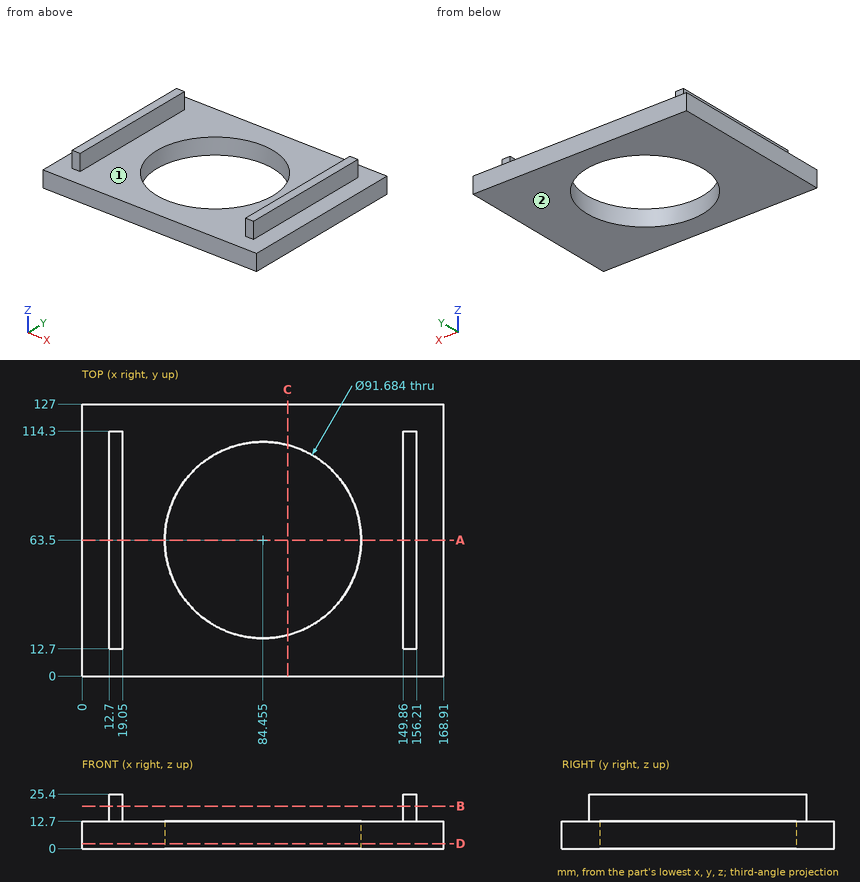
Can you work these out from the drawing? Everything is in mm from the part's minimum corner. Coordinates: 2 decimals unless noted, no trailing zeros. Write each loop counter-clockwise with the first axis right and the second up, starting at its lowest first coordinate (ties: lowest second). Pieces come first, ordered by that corner, then holes. Notation, with made-up numbers: (-13, 9.5) -> (38, 9.5) arc R27 cw to (38, 30.5) -> close; hole circle Ø4 at (21, 87.5). An arc over 180 degrees is marked (long way). Write item = value, one per line.
(1) For pin 1 (12 mm diameter, centred on y = 103.5, z = 18, fed in from +X); pin 2 (7 mm diameter, centred on x = 152.5, z = 22, fed in from -Y); pin 3 (3 mm diameter, centred on x = 154, z = 21.5, fed in from +Y); pin 4 (4 mm diameter, centred on x = 79, y = 21, fed in from -Z), each with a flat end and sliding along its axis, tell me the tip position at first contact or that it passes through.
Verdict:
pin_1 = 168.91
pin_2 = 12.7
pin_3 = 114.3
pin_4 = through
(2) Imagine slicing it at C-C (x = 96). Please give me the cut outline in (y, z).
Verdict:
outline = (0, 0) -> (19.14, 0) -> (19.14, 12.7) -> (0, 12.7) -> close; (107.86, 0) -> (127, 0) -> (127, 12.7) -> (107.86, 12.7) -> close
(3) Imagine slicing it at D-D (z = 2.25). Please give me the cut outline in (x, y) (1 decimal).
Verdict:
outline = (0, 0) -> (168.9, 0) -> (168.9, 127) -> (0, 127) -> close; hole circle Ø91.7 at (84.5, 63.5)
(4) If I drill on probe 1 along X at (y, z) = (63.5, 8.25); probe 2 along X at (y, z) = (33, 24.25); probe 3 along Y at (x, z) = (16.5, 16.5), over which ranges is the centre line in solid material (lowest first)?
Verdict:
probe_1 = 0 to 38.61, 130.3 to 168.91
probe_2 = 12.7 to 19.05, 149.86 to 156.21
probe_3 = 12.7 to 114.3
(5) Thinking about a two-plate mould opening in X: for the marked faces 1 and 2, which applies, +X half, -X half, draft (parallel to the pull), parting line (faces both ways), or undercut?
Verdict:
face_1 = undercut
face_2 = draft
(6) Imagine slicing it at A-A (y = 63.5). Please give me the cut outline in (x, z), and give its area (3 significant figures).
Verdict:
outline = (0, 0) -> (38.61, 0) -> (38.61, 12.7) -> (19.05, 12.7) -> (19.05, 25.4) -> (12.7, 25.4) -> (12.7, 12.7) -> (0, 12.7) -> close; (130.3, 0) -> (168.91, 0) -> (168.91, 12.7) -> (156.21, 12.7) -> (156.21, 25.4) -> (149.86, 25.4) -> (149.86, 12.7) -> (130.3, 12.7) -> close
area = 1,140 mm^2
(7) Imagine slicing it at B-B (z = 19.75). Please give me the cut outline in (x, y).
Verdict:
outline = (12.7, 12.7) -> (19.05, 12.7) -> (19.05, 114.3) -> (12.7, 114.3) -> close; (149.86, 12.7) -> (156.21, 12.7) -> (156.21, 114.3) -> (149.86, 114.3) -> close
